```python
from build123d import *
from build123d.topology import SkipClean

# Parameters (mm, degrees)
SKETCH1_R           = 18.5
BOSS_EXTRUDE1_DEPTH = 23
SKETCH2_R           = 10.95
BOSS_EXTRUDE2_DEPTH = 3.5
SKETCH4_R           = 3.05
CUT_EXTRUDE1_DEPTH  = 4.1
SKETCH5_R           = 1.5
CUT_EXTRUDE2_DEPTH  = 4
SKETCH7_R           = 10.95
SKETCH7_R_2         = 3
BOSS_EXTRUDE3_DEPTH = 11
SKETCH9_R           = 1.5
CUT_EXTRUDE4_DEPTH  = 46.724719791
SKETCH10_R          = 3
CUT_EXTRUDE5_DEPTH  = 46.724719791
SKETCH11_R          = 3.25
CUT_EXTRUDE8_DEPTH  = 30
BOSS_EXTRUDE4_START = 7
SKETCH12_R          = 18.5
SKETCH12_R_2        = 3.25
SKETCH12_R_3        = 3.05
BOSS_EXTRUDE4_DEPTH = 7
CUT_EXTRUDE9_START  = -5
SKETCH13_R          = 1.5
CUT_EXTRUDE9_DEPTH  = 17
CIRPATTERN1_COUNT   = 3


with BuildPart() as part:
    # Sketch1 → Boss-Extrude1 (new body)
    with BuildSketch(Plane.XY):
        Circle(SKETCH1_R)
    extrude(amount=BOSS_EXTRUDE1_DEPTH)

    # Sketch2 → Boss-Extrude2 (add)
    with BuildSketch(Plane.XY.offset(23)):
        Circle(SKETCH2_R)
    extrude(amount=BOSS_EXTRUDE2_DEPTH)

    # Sketch4 → Cut-Extrude1 (cut)
    with BuildSketch(Plane(origin=(0, 0, 0), x_dir=(-1, 0, 0), z_dir=(0, 0, -1))):
        Circle(SKETCH4_R)
    extrude(amount=-CUT_EXTRUDE1_DEPTH, mode=Mode.SUBTRACT)

    # Sketch5 → Cut-Extrude2 (cut)
    with BuildSketch(Plane(origin=(0, 0, 4.1), x_dir=(-1, 0, 0), z_dir=(0, 0, -1))):
        Circle(SKETCH5_R)
    extrude(amount=-CUT_EXTRUDE2_DEPTH, mode=Mode.SUBTRACT)

    # Sketch7 → Boss-Extrude3 (add)
    with BuildSketch(Plane.XY.offset(26.5)):
        Circle(SKETCH7_R)
        Circle(SKETCH7_R_2, mode=Mode.SUBTRACT)
    extrude(amount=BOSS_EXTRUDE3_DEPTH)

    # Sketch9 → Cut-Extrude4 (cut, through all)
    with BuildSketch(Plane.XY.offset(37.5)):
        with Locations((7, 0)):
            Circle(SKETCH9_R)
        with Locations((-3.5, -6.062177826)):
            Circle(SKETCH9_R)
        with Locations((-3.5, 6.062177826)):
            Circle(SKETCH9_R)
    extrude(amount=-CUT_EXTRUDE4_DEPTH, mode=Mode.SUBTRACT)

    # Sketch10 → Cut-Extrude5 (cut, through all)
    with SkipClean():  # the faces are left unmerged after this step: merging them gives an invalid solid
        with BuildSketch(Plane.XY.offset(37.5)):
            with Locations(Location((0, 0, 0), (0, 0, 180))):
                Circle(SKETCH10_R)
        extrude(amount=-CUT_EXTRUDE5_DEPTH, mode=Mode.SUBTRACT)

    # Sketch11 → Cut-Extrude8 (cut)
    with SkipClean():  # the faces are left unmerged after this step: merging them gives an invalid solid
        with BuildSketch(Plane(origin=(0, 0, 0), x_dir=(-1, 0, 0), z_dir=(0, 0, -1))):
            with Locations((3.5, -6.062177826)):
                Circle(SKETCH11_R)
            with Locations((3.5, 6.062177826)):
                Circle(SKETCH11_R)
            with Locations((-7, 0)):
                Circle(SKETCH11_R)
        extrude(amount=-CUT_EXTRUDE8_DEPTH, mode=Mode.SUBTRACT)
    add(part.part.scale(1), mode=Mode.REPLACE)  # the faces are merged on a copy

    # Sketch12 → Boss-Extrude4 (add)
    with BuildSketch(Plane(origin=(0, 0, 0), x_dir=(-1, 0, 0), z_dir=(0, 0, -1)).offset(BOSS_EXTRUDE4_START)):
        Circle(SKETCH12_R)
        with Locations((3.5, 6.062177826)):
            Circle(SKETCH12_R_2, mode=Mode.SUBTRACT)
        with Locations((3.5, -6.062177826)):
            Circle(SKETCH12_R_2, mode=Mode.SUBTRACT)
        with Locations((-7, 0)):
            Circle(SKETCH12_R_2, mode=Mode.SUBTRACT)
        Circle(SKETCH12_R_3, mode=Mode.SUBTRACT)
    extrude(amount=-BOSS_EXTRUDE4_DEPTH)

    # Sketch13 → Cut-Extrude9 (cut)
    with BuildSketch(Plane(origin=(0, 0, 0), x_dir=(0, 0, -1), z_dir=(1, 0, 0)).offset(CUT_EXTRUDE9_START)):
        with Locations((2, 0)):
            Circle(SKETCH13_R)
    cut_extrude9 = extrude(amount=-CUT_EXTRUDE9_DEPTH, mode=Mode.SUBTRACT)

    # CirPattern1: Cut-Extrude9 ×3 about axis
    cirpattern1_axis = Axis((0, 0, 0), (0, 0, 1))
    for i in range(1, CIRPATTERN1_COUNT):
        add(cut_extrude9.rotate(cirpattern1_axis, i * 360 / CIRPATTERN1_COUNT), mode=Mode.SUBTRACT)


solid = part.part
```
Model file for the job. Use its own axes, mm. A direction names the side the tool comes from. Round coordinates to 2 decimals unless told otherwise and drop trailing zeros. Write each loop counter-clockwise with the first axis right and the second up, starting at its lowest first coordinate (ties: lowest second). Pieces come first, ordered by that corner, then holes. Notation, with made-up numbers: M 21.25,33 L 32.25,33 A30 cw 32.25,57 Z; hole C 2,30 d10. An arc over 180 degrees is marked long. Put each result on its own line as item: value.
Item 1: Cut at B-B (x = -10). List the corners of the cut face in (y, z).
Responses:
outline: M -15.56,-7 L 15.56,-7 L 15.56,23 L 4.46,23 L 4.46,37.5 L -4.46,37.5 L -4.46,23 L -15.56,23 Z; hole C 0,-2 d3
Item 2: Flat gauge pins, fed straight in: P1, Ø10, axis at y = 9.5, z = 16.5, coming from the +X side; P2, Ø4, axis at y = 11, z = 27.5, coming from the -X side; P3, Ø1.5, axis at y = 8.5, z = 17.5, coming from the -X side; P4, Ø2.5, axis at x = -3.5, y = 6.06, coming from the -Z side (3 decimals). Where does each tip first touch, or does it go through?
Responses:
P1: x = 17.94
P2: x = -6.24
P3: x = -16.8
P4: through
Item 3: Cut at C-C (x = 0.5). List the corners of the cut face in (y, z), and give its area (3 significant figures).
Responses:
outline: M -18.49,-7 L -3.01,-7 L -3.01,4.1 L -2.96,4.1 L -2.96,37.5 L -10.94,37.5 L -10.94,23 L -18.49,23 Z; M 2.96,4.1 L 3.01,4.1 L 3.01,-7 L 18.49,-7 L 18.49,23 L 10.94,23 L 10.94,37.5 L 2.96,37.5 Z
area: 1,160 mm²
Item 4: Mould opens along Z. For faces 4 (the flat face through (-5, 5, 30)), 5 (the cylindrical face through (-2.1, -6.6, 33.8)), 6 (the flat face through (-5, 0, -2)) say: +Z half, -Z half, draft (parallel to the pull), parting line (faces both ways), or undercut.
Responses:
face 4: -Z half
face 5: draft
face 6: undercut
Item 5: Cut at A-A (z = -2). List the corners of the cut face in (x, y).
Responses:
outline: M -18.44,-1.5 A18.5 ccw 7.92,-16.72 L 1.2,-5.08 L 3.8,-3.58 L 10.52,-15.22 A18.5 ccw 10.52,15.22 L 3.8,3.58 L 1.2,5.08 L 7.92,16.72 A18.5 ccw -18.44,1.5 L -5,1.5 L -5,-1.5 Z; hole C -3.5,-6.06 d6.5; hole C -3.5,6.06 d6.5; hole C 0,0 d6.1; hole C 7,0 d6.5
Item 6: Tool access for faces 1 (the flat face through (8, -8, 23)), 2 (the flat face through (2.52, 4.32, -1.98)), 3 (the flat face through (-5, -7, 30)): list every direction of +Z, -Z, +X, -X, +Y, -Y with a clear straight run to the whole face (end or side of a thin tool).
Responses:
face 1: +Z
face 2: none
face 3: -Z
Item 7: Cut at D-D (x = 7). State how many separate pieces and enclosed holes the cut face has, and give its area (3 significant figures).
Responses:
separate pieces: 2
enclosed holes: 2
area: 980 mm²
Item 8: Probe L1, parallel to Y at x = -3.5, z = 15.5; L2, parallel to X at y = 2.5, z = 3.5; L3, parallel to Z at x = -4, y = 3.5. List the from-to ranges inside material, lowest first. Write a range as from..to.
Responses:
L1: -18.17..-9.31, -2.81..2.81, 9.31..18.17
L2: -18.33..-1.75, 1.75..4.92, 9.08..18.33
L3: 30..37.5
